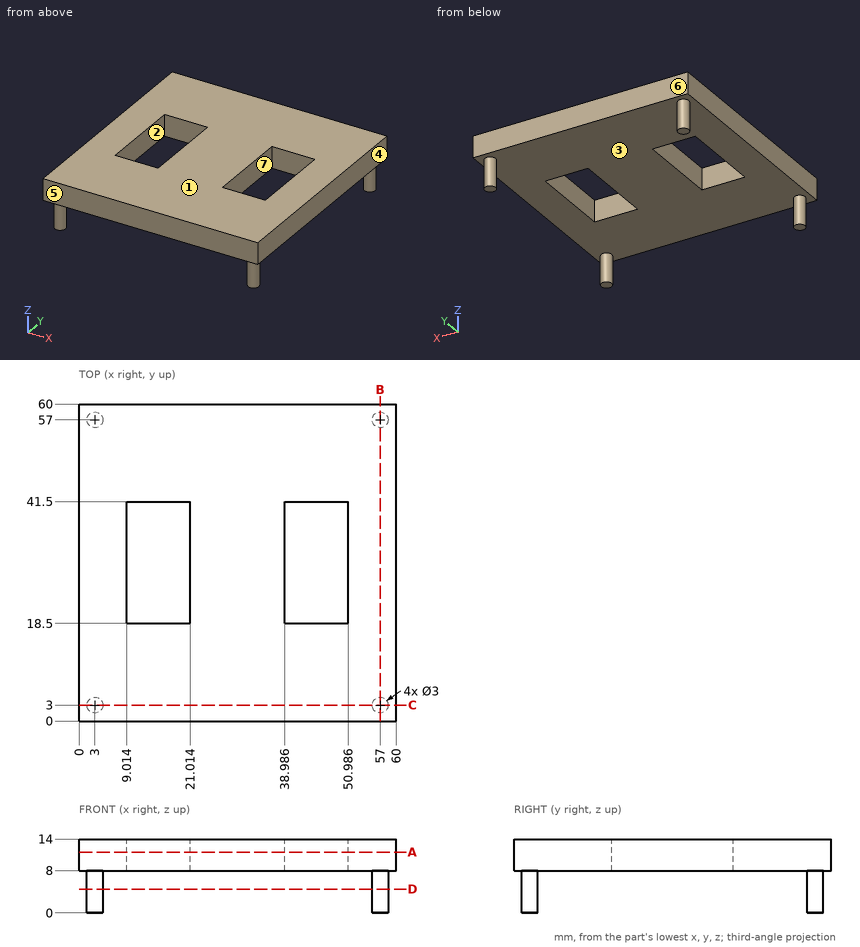
Source: three-view drawing plus pictorial views. Frame: mm from the lowest corner of the part. A direction names the side the tool comes from. Coordinates: 2 decimals unless noted, no trailing zeros. Order: outer loops, then holes, each group sorted by start corner. A loop starts at its lowest first (then second) coordinate and runs counter-clockwise, first axis right, second up.
1) First-contact query: P1, Ø8, axis at x = 51.5, y = 18, coming from the -Z side; P2, Ø5, axis at y = 29.5, z = 12, coming from the -X side. Flat tips, straight axial feed; report the tip coordinate or a pass-through.
Result sheet:
P1: stops at z = 8
P2: stops at x = 0
2) Section D-D (z = 4.5). Return loops of the section in (x, y).
Result sheet:
outline: circle Ø3 at (3, 3); circle Ø3 at (3, 57); circle Ø3 at (57, 3); circle Ø3 at (57, 57)
3) Section A-A (z = 11.5). Return loops of the section in (x, y) (1 decimal), then the cut area to 3 significant figures.
Result sheet:
outline: (0, 0) - (60, 0) - (60, 60) - (0, 60) - close; hole (9, 18.5) - (21, 18.5) - (21, 41.5) - (9, 41.5) - close; hole (39, 18.5) - (51, 18.5) - (51, 41.5) - (39, 41.5) - close
area: 3,050 mm2
4) Section B-B (x = 57). Return loops of the section in (y, z), then the cut area to 3 significant figures.
Result sheet:
outline: (0, 8) - (1.5, 8) - (1.5, 0) - (4.5, 0) - (4.5, 8) - (55.5, 8) - (55.5, 0) - (58.5, 0) - (58.5, 8) - (60, 8) - (60, 14) - (0, 14) - close
area: 408 mm2
5) Set-up query: the marked faces 1, 2 and 3. Return all of +Z, -Z, +X, -X, +Y, -Y with unobstructed straight access to the full face (end or side cutting, diameter ignored); none if empty.
Result sheet:
face 1: +Z, +X, -X, +Y, -Y
face 2: +Z, -Z
face 3: -Z
6) Draft query along Y for the marked faces 4, 5, 6 and 7. Return one class per face: released by +Y, released by -Y, zero draft, split by the parting line, or undercut.
Result sheet:
face 4: zero draft
face 5: released by -Y
face 6: released by +Y
face 7: undercut
7) Ray query, probe 1 along X at (y, z) = (37.5, 12.75) (1 decimal); probe 2 along Y at (x, z) = (44.5, 11.25); probe 3 along Y at (x, z) = (3, 5.25). Return the intervals inside material, ascending.
Result sheet:
probe 1: x = 0 to 9, 21 to 39, 51 to 60
probe 2: y = 0 to 18.5, 41.5 to 60
probe 3: y = 1.5 to 4.5, 55.5 to 58.5
